Check sheet for the modelled part. Datum: model origin and axes. Units: mm. A direction names the side the tool comes from. Round coordinates to 2 decimals unless told otherwise and drop trailing zeros. Order: outer loops, then holes, each group sorted by start corner. A loop starts at its lowest first (then second) coordinate and runs counter-clockwise, first axis right, second up.
```python
from build123d import *

# Parameters (mm, degrees)
EXTRUDE_1_DEPTH = 3.375
FILLET_1_R      = 1
SKETCH_3_R      = 3
EXTRUDE_2_DEPTH = 21


with BuildPart() as part:
    # 草图1 → 凸台-拉伸1 (new body, symmetric)
    with BuildSketch(Plane(origin=(0, 0, 0), x_dir=(1, 0, 0), z_dir=(0, 1, 0))):
        with BuildLine():
            Line((-3, -15), (3, -15))
            Line((3, -15), (8.702459553, -4.926174756))
            ThreePointArc((8.702459553, -4.926174756), (0, 10), (-8.702459553, -4.926174756))
            Line((-8.702459553, -4.926174756), (-3, -15))
        make_face()
    extrude(amount=EXTRUDE_1_DEPTH, both=True)

    # 草图2 → 切除-旋转1 (revolve, cut)
    with BuildSketch(Plane(origin=(0, 0, 0), x_dir=(0, 0, -1), z_dir=(1, 0, 0))):
        with BuildLine():
            Line((0, 6.35), (0, -6.35))
            ThreePointArc((0, -6.35), (6.35, 0), (0, 6.35))
        make_face()
    revolve(axis=Axis((0, 6.35, 0), (0, -1, 0)), mode=Mode.SUBTRACT)

    # 圆角1
    fillet_1_edges = [part.edges().sort_by_distance(p)[0] for p in [
        (5.851229777, 3.375, 9.963087378),
        (0, 3.375, -10),
        (-5.851229777, 3.375, 9.963087378),
        (0, -3.375, -10),
        (5.851229777, -3.375, 9.963087378),
        (-5.851229777, -3.375, 9.963087378),
    ]]
    fillet(fillet_1_edges, radius=FILLET_1_R)

    # 草图3 → 凸台-拉伸2 (add)
    with BuildSketch(Plane.XY.offset(15)):
        Circle(SKETCH_3_R)
    extrude(amount=EXTRUDE_2_DEPTH)


solid = part.part
```
Item 1: Go/stop test with flat-tipped pins: P1, Ø3, axis at y = 0.5, z = 20.5, coming from the +X side; P2, Ø4, axis at x = 4.5, y = -2.5, coming from the +Z side; P3, Ø8, axis at x = 5.5, z = 26.5, coming from the +Y side. Record where each tip stops, or that it passes through.
Answer:
P1: stops at x = 3
P2: stops at z = 15
P3: stops at y = 2.6
Item 2: Sectioned sample at A-A (y = -0.5). Record the cut outline in (x, z), and give its area (3 significant figures).
Answer:
outline: (-8.7, 4.93) arc R10 ccw (long way) to (8.7, 4.93) - (3, 15) - (2.96, 15) - (2.96, 36) - (-2.96, 36) - (-2.96, 15) - (-3, 15) - close; hole circle Ø12.66 at (0, 0)
area: 368 mm2
Item 3: Access from +Z, -Z, +X, -X, +Y, -Y to the whole of each face (thin tool, end or side, straight path). Record for faces 1 (the flat face through (-0.2, 3.2, 15)), 2 (the flat face through (0.2, -3.2, 15)), 3 (the cylindrical face through (-3, 0, 25)).
Answer:
face 1: +Z, +Y
face 2: +Z, -Y
face 3: +Z
Item 4: Sectioned sample at C-C (z = 30). Record the cut outline in (x, y).
Answer:
outline: circle Ø6 at (0, 0)
Item 5: Sectioned sample at D-D (y = 1.75). Record the cut outline in (x, z).
Answer:
outline: (-8.7, 4.93) arc R10 ccw (long way) to (8.7, 4.93) - (3, 15) - (2.44, 15) - (2.44, 36) - (-2.44, 36) - (-2.44, 15) - (-3, 15) - close; hole circle Ø12.21 at (0, 0)
Item 6: Scan lines: line 1 along Z through (x, y) = (3.25, -0.75); line 2 along X through (y, z) = (-2.5, 3); line 3 along X through (y, z) = (0.25, 2.5). Record each from-to range of solid material in increasing order.
Answer:
line 1: z = -9.46 to -5.4, 5.4 to 14.56
line 2: x = -9.53 to -5.01, 5.01 to 9.53
line 3: x = -9.68 to -5.83, 5.83 to 9.68
Item 7: Sectioned sample at B-B (x = 0). Record the cut outline in (y, z) (3 decimals).
Answer:
outline: (-3.375, -9) arc R1 ccw to (-2.375, -10) - (2.375, -10) arc R1 ccw to (3.375, -9) - (3.375, -5.379) arc R6.35 cw to (-3.375, -5.379) - close; (-3.375, 5.379) arc R6.35 cw to (3.375, 5.379) - (3.375, 15) - (3, 15) - (3, 36) - (-3, 36) - (-3, 15) - (-3.375, 15) - close
